Design review of the part built by this model. Coordinates are the model's own, in mm. A direction names the side the tool comes from. Round coordinates to 2 decimals unless told otherwise and drop trailing zeros. Order: outer loops, then holes, each group sorted by start corner. A loop starts at its lowest first (then second) coordinate and runs counter-clockwise, first axis right, second up.
from build123d import *

# Parameters (mm, degrees)
F1_DEPTH      = 1.32842
F2_R          = 6.858
F3_DEPTH      = 1.32942
F3_DEPTH_BACK = 1.32942
F5_DEPTH      = 2.65784


with BuildPart() as f1:
    # F0 (on Right) → F1 (new body, symmetric)
    with BuildSketch(Plane.YZ):
        with BuildLine():
            Line((0, 31.3182), (-9.525, 31.3182))
            Line((-9.525, 31.3182), (-9.525, -21.7932))
            ThreePointArc((-9.525, -21.7932), (-6.7351920908, -28.5283920908), (0, -31.3182))
            Line((0, -31.3182), (9.525, -31.3182))
            Line((9.525, -31.3182), (9.525, 21.7932))
            ThreePointArc((9.525, 21.7932), (6.7351920908, 28.5283920908), (0, 31.3182))
        make_face()
    extrude(amount=F1_DEPTH, both=True)

    # F2 (on Right) → F3 (cut, two sides)
    with BuildSketch(Plane.YZ) as f3_sk:
        Circle(F2_R)
    extrude(amount=-F3_DEPTH, mode=Mode.SUBTRACT)
    extrude(f3_sk.sketch, amount=F3_DEPTH_BACK, mode=Mode.SUBTRACT)

    # F4 (on face) → F5 (cut, through all)
    with BuildSketch(Plane(origin=(-1.32842, 0, 0), x_dir=(0, -1, 0), z_dir=(-1, 0, 0))):
        with BuildLine():
            Line((2.794, 20.6397468008), (2.794, 22.8165670731))
            ThreePointArc((2.794, 22.8165670731), (0, 22.987), (-2.794, 22.8165670731))
            Line((-2.794, 22.8165670731), (-2.794, 20.6397468008))
            ThreePointArc((-2.794, 20.6397468008), (0, 20.828), (2.794, 20.6397468008))
        make_face()
        with BuildLine():
            Line((-2.794, -20.6397468008), (-2.794, -22.8165670731))
            ThreePointArc((-2.794, -22.8165670731), (0, -22.987), (2.794, -22.8165670731))
            Line((2.794, -22.8165670731), (2.794, -20.6397468008))
            ThreePointArc((2.794, -20.6397468008), (0, -20.828), (-2.794, -20.6397468008))
        make_face()
    extrude(amount=-F5_DEPTH, mode=Mode.SUBTRACT)


solid = f1.part
1) Take a section at B-B on z = 0. Give the boundary of the cut face in (x, y) (3 decimals), plus the area to 3 significant figures.
Results:
outline: (-1.328, -9.525) - (1.328, -9.525) - (1.328, -6.858) - (-1.328, -6.858) - close; (-1.328, 6.858) - (1.328, 6.858) - (1.328, 9.525) - (-1.328, 9.525) - close
area: 14.2 mm2
2) The part is to be moulded in two halves that separate along Y. For faces 3 (the face through (0, -9.525, 5)), 4 (the face through (0, -5, 31.318)), 5 (the face through (-0.019, -0.039, 22.987)), say which applies: released by +Y, released by -Y, zero draft, split by the parting line, or undercut.
Results:
face 3: released by -Y
face 4: zero draft
face 5: undercut
3) For faces 1 (the face through (0, 2.794, -22)), 2 (the face through (0.02, -6.81, -28.45)), list the 3-axis set-ups (+Z, -Z, +X, -X, +Y, -Y) from which the entire face can be reached by the end or side of a thin tool; tool diameter is ignored.
Results:
face 1: +X, -X
face 2: -Z, +X, -X, -Y
4) Take a section at C-C on y = 5.5. Give the boundary of the cut face in (x, z), plus the area to 3 significant figures.
Results:
outline: (-1.33, -31.32) - (1.33, -31.32) - (1.33, -4.1) - (-1.33, -4.1) - close; (-1.33, 4.1) - (1.33, 4.1) - (1.33, 29.57) - (-1.33, 29.57) - close
area: 140 mm2
5) Take a section at A-A on x = -0.2. Give the boundary of the cut face in (y, z) (3 decimals).
Results:
outline: (-9.525, -21.793) arc R9.525 ccw to (0, -31.318) - (9.525, -31.318) - (9.525, 21.793) arc R9.525 ccw to (0, 31.318) - (-9.525, 31.318) - close; hole circle Ø13.716 at (0, 0); hole (-2.794, -22.817) arc R22.987 ccw to (2.794, -22.817) - (2.794, -20.64) arc R20.828 cw to (-2.794, -20.64) - close; hole (-2.794, 20.64) arc R20.828 cw to (2.794, 20.64) - (2.794, 22.817) arc R22.987 ccw to (-2.794, 22.817) - close
6) Clearance check with a flat-ended pin moving along its axis: P1, Ø11, axis at y = 0, z = 0, coming from the -X side. State where the tip first meets the part, or that it passes through.
Results:
P1: passes through
7) To check wall thickness, follow line 1 along Z through (x, y) = (1.2, -0.5); line 2 along Y through (x, z) = (0.45, 0) (3 decimals); line 3 along Z through (x, y) = (1.15, -2.25). State the ranges of each line that lie inside material, in increasing order.
Results:
line 1: z = -31.31 to -22.98, -20.82 to -6.84, 6.84 to 20.82, 22.98 to 31.32
line 2: y = -9.525 to -6.858, 6.858 to 9.525
line 3: z = -31.05 to -22.88, -20.71 to -6.48, 6.48 to 20.71, 22.88 to 31.32
8) Take a section at D-D on y = -2. Give the boundary of the cut face in (x, z), plus the area to 3 significant figures.
Results:
outline: (-1.33, -31.11) - (1.33, -31.11) - (1.33, -22.9) - (-1.33, -22.9) - close; (-1.33, -20.73) - (1.33, -20.73) - (1.33, -6.56) - (-1.33, -6.56) - close; (-1.33, 6.56) - (1.33, 6.56) - (1.33, 20.73) - (-1.33, 20.73) - close; (-1.33, 22.9) - (1.33, 22.9) - (1.33, 31.32) - (-1.33, 31.32) - close
area: 119 mm2
